Autodesk Fusion 360 part; units mm, degrees
sketch "Sketch1" plane through (0, 0, 0) normal (0, 1, 0) x (1, 0, 0)
  line L0 (0, 0) -> (55, 0)
  line L1 (0, 0) -> (0, 110)
  line L2 (0, 110) -> (55, 110)
  line L3 (55, 110) -> (55, 94.5)
  line L4 (55, 94.5) -> (8, 94.5)
  line L5 (8, 94.5) -> (8, 15.5)
  line L6 (8, 15.5) -> (55, 15.5)
  line L7 (55, 15.5) -> (55, 0)
  line L8 (55, 15.5) -> (55, 22.5)
  line L9 (55, 22.5) -> (15, 22.5)
  line L10 (15, 22.5) -> (15, 87.5)
  line L11 (15, 87.5) -> (55, 87.5)
  line L12 (55, 87.5) -> (55, 94.5)
  line L13 (4, 0) -> (4, 110) construction
  circle A0 centre (51, 7.5) radius 1.55
  circle A1 centre (4, 7.5) radius 1.55
  circle A2 centre (4, 102.5) radius 1.55
  circle A3 centre (51, 102.5) radius 1.55
  circle A4 centre (4, 70.84) radius 1.55
  circle A5 centre (4, 39.16) radius 1.55
  line L14 (52.55, 4.5) -> (52.55, 10.5)
  arc A6 (52.55, 10.5) -> (49.45, 10.5) centre (51, 10.5) ccw
  line L15 (49.45, 10.5) -> (49.45, 4.5)
  arc A7 (49.45, 4.5) -> (52.55, 4.5) centre (51, 4.5) ccw
  line L16 (51, 4.5) -> (51, 10.5) construction
  line L17 (51, 99.5) -> (51, 105.5) construction
  line L18 (5.55, 99.5) -> (5.55, 105.5)
  arc A8 (5.55, 105.5) -> (2.45, 105.5) centre (4, 105.5) ccw
  line L19 (2.45, 105.5) -> (2.45, 99.5)
  arc A9 (2.45, 99.5) -> (5.55, 99.5) centre (4, 99.5) ccw
  line L20 (4, 99.5) -> (4, 105.5) construction
  line L21 (52.55, 99.5) -> (52.55, 105.5)
  arc A10 (52.55, 105.5) -> (49.45, 105.5) centre (51, 105.5) ccw
  line L22 (49.45, 105.5) -> (49.45, 99.5)
  arc A11 (49.45, 99.5) -> (52.55, 99.5) centre (51, 99.5) ccw
  line L23 (51, 99.5) -> (51, 105.5) construction
  line L24 (5.55, 4.5) -> (5.55, 10.5)
  arc A12 (5.55, 10.5) -> (2.45, 10.5) centre (4, 10.5) ccw
  line L25 (2.45, 10.5) -> (2.45, 4.5)
  arc A13 (2.45, 4.5) -> (5.55, 4.5) centre (4, 4.5) ccw
  line L26 (4, 4.5) -> (4, 10.5) construction
  point P0 (51, 7.5)
  point P1 (51, 102.5)
  point P2 (4, 102.5)
  point P3 (51, 102.5)
  point P4 (4, 7.5)
  dimension "d1" = 65
  dimension "d2" = 7
  dimension "d3" = 15.5
  dimension "d4" = 7
  dimension "d5" = 8
  dimension "d7" = 40
  dimension "d8" = 4
  dimension "d9" = 3.1
  dimension "d10" = 3.1
  dimension "d11" = 3.1
  dimension "d12" = 3.1
  dimension "d14" = 4
  dimension "d15" = 4
  dimension "d34" = 7.5
  dimension "d35" = 7.5
  dimension "d36" = 7.5
  dimension "d37" = 7.5
  dimension "d38" = 3.1
  dimension "d39" = 3.1
  dimension "d40" = 31.66
  dimension "d41" = 31.66
  dimension "d42" = 3.1
  dimension "d43" = 3.1
  dimension "d44" = 3.1
  dimension "d45" = 3.1
  dimension "d46" = 3
  dimension "d47" = 3
  dimension "d48" = 3
  dimension "d49" = 3
extrude "Extrude1" add sketch "Sketch1" along normal blind 4 contours L0 L1 L2 L3 L4 L5 L6 L7
extrude "Extrude2" add sketch "Sketch1" along normal blind 40 contours L4 L5 L6 L8 L9 L10 L11 L12
fillet "Fillet1" radius 3 6 edges at (55, 2, 0) (8, 22, -15.5) (0, 2, 0) (55, 2, -110) (8, 22, -94.5) (0, 2, -110)
fillet "Fillet1" radius 3 2 edges at (55, 22, -94.5) (55, 22, -15.5)
equation "d4 = d2"
equation "d10 = d9"
equation "d15 = d14"
equation "d42 = d9"
equation "d43 = d9"
equation "d44 = d9"
equation "d45 = d9"
equation "d47 = d46"
equation "d48 = d46"
equation "d49 = d46"
CAD build for the part. Positions are in the model's coordinates, mm. A direction names the side the tool comes from. Give positions to 0.01 mm unless a question says otherwise; leave off trailing zeros. Loops run counter-clockwise (first coordinate to the right, second up) from the corner with the lowest first, then second, coordinate; pieces in that order, holes last. Notation, with made-up numbers: M -9,8 L 21,8 A17 cw 21,18 Z; hole C -2.5,-6 d8. An arc over 180 degrees is marked long. Answer in a Markdown table with one row per item. Add a question column.
Item 1: Mould opens along X. For faces 1 (the face through (2.86, 1.97, -38.11)), 2 (the face through (27, 2, -110)), 3 (the face through (55, 14, -91)) say: +X half, -X half, draft (parallel to the pull), parting line (faces both ways), or undercut.
Item 2: Drop flat-ended pins along their axis: P1, Ø1, axis at x = 15.5, y = 23, coming from the -Z side; P2, Ø3.5, axis at x = 4, z = -70.84, coming from the +Y side; P3, Ø10, axis at y = 23, z = -15, coming from the -X side. Give the stop position or say it passes through.
Item 3: Band-saw the part on C-C on z = -9. Give the cut face in (x, y).
Item 4: Probe probe 1 along Z at (x, y) = (4, 3.15); probe 2 along Z at (x, y) = (47.5, 17); probe 3 along X at (y, z) = (2, -39). List the from-to ranges inside material, lowest first.
Item 5: Tool access for faces 4 (the face through (15, 20, -55)), 5 (the face through (27, 2, 0)), 6 (the face through (5.55, 2, -102)): list every direction of +Z, -Z, +X, -X, +Y, -Y with a clear straight run to the whole face (end or side of a thin tool).
Item 6: Band-saw the part on A-A on x = 29. Give the cut face in (y, z).
Item 7: Band-saw the part on B-B on z = -39.16. Give the cut face in (x, y), then the cut area to 3 significant figures.
Item 8: Band-saw the part on D-D on y = 35. Give the cut face in (x, z).
Reply:
| question | item | result |
|---|---|---|
| 1 | face 1 | undercut |
| 1 | face 2 | draft |
| 1 | face 3 | +X half |
| 2 | P1 | stops at z = -94.5 |
| 2 | P2 | stops at y = 4 |
| 2 | P3 | stops at x = 8 |
| 3 | outline | M 0,0 L 2.45,0 L 2.45,4 L 0,4 Z; M 5.55,0 L 49.45,0 L 49.45,4 L 5.55,4 Z; M 52.55,0 L 55,0 L 55,4 L 52.55,4 Z |
| 4 | probe 1 | z = -110 to -107.05, -97.95 to -72.39, -69.29 to -40.71, -37.61 to -12.05, -2.95 to 0 |
| 4 | probe 2 | z = -94.5 to -87.5, -22.5 to -15.5 |
| 4 | probe 3 | x = 0 to 2.46, 5.54 to 15 |
| 5 | face 4 | +X, +Y, -Y |
| 5 | face 5 | +Z, +X, -X, +Y, -Y |
| 5 | face 6 | +Y, -Y |
| 6 | outline | M 0,-110 L 4,-110 L 4,-94.5 L 40,-94.5 L 40,-87.5 L 0,-87.5 Z; M 0,-22.5 L 40,-22.5 L 40,-15.5 L 4,-15.5 L 4,0 L 0,0 Z |
| 7 | outline | M 0,0 L 2.45,0 L 2.45,4 L 0,4 Z; M 5.55,0 L 15,0 L 15,40 L 8,40 L 8,4 L 5.55,4 Z |
| 7 | area | 300 mm^2 |
| 8 | outline | M 8,-91.5 A3 ccw 11,-94.5 L 52,-94.5 A3 ccw 55,-91.5 L 55,-87.5 L 15,-87.5 L 15,-22.5 L 55,-22.5 L 55,-18.5 A3 ccw 52,-15.5 L 11,-15.5 A3 ccw 8,-18.5 Z |
